Source: CAD feature listing. Evaluate the final solid. Frame: model axes, mm. Round coordinates to 2 decimals unless told otherwise and drop trailing zeros. Write each loop counter-clockwise with the first axis right and the second up, starting at its lowest first coordinate (ties: lowest second). Pieces come first, ordered by that corner, then holes. Notation, with made-up numbers: M 69.25,0.25 L 91.25,0.25 A25 ccw 91.25,27.25 Z; hole C 49.5,77 d8. An arc over 180 degrees is marked long. Use a Markdown table: item, result.
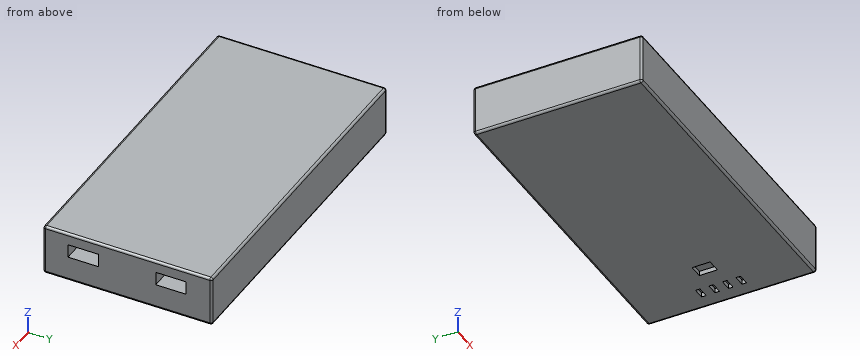
```python
from build123d import *

# Parameters (mm, degrees)
SKETCH_W        = 145
SKETCH_H        = 75
PAD_DEPTH       = 22.5
FILLET_R        = 1
SKETCH001_W     = 5
SKETCH001_H     = 2
SKETCH001_W_2   = 6
SKETCH001_H_2   = 8
POCKET_DEPTH    = 2
SKETCH002_W     = 13.5
SKETCH002_H     = 6
POCKET001_DEPTH = 20


with BuildPart() as part:
    # Sketch → Pad (new body)
    with BuildSketch(Plane.XY):
        Rectangle(SKETCH_W, SKETCH_H)
    extrude(amount=PAD_DEPTH)

    # Fillet
    fillet_edges = [part.edges().sort_by_distance(p)[0] for p in [
        (0, -37.5, 22.5),
        (72.5, 0, 22.5),
        (0, 37.5, 22.5),
        (-72.5, 0, 22.5),
        (-72.5, -37.5, 11.25),
        (72.5, -37.5, 11.25),
        (72.5, 37.5, 11.25),
        (72.5, 0, 0),
        (0, -37.5, 0),
        (0, 37.5, 0),
        (-72.5, 0, 0),
        (-72.5, 37.5, 11.25),
    ]]
    fillet(fillet_edges, radius=FILLET_R)

    # Sketch001 (on Face13 of Fillet) → Pocket (cut)
    with BuildSketch(Plane(origin=(0, 0, 0), x_dir=(1, 0, 0), z_dir=(0, 0, -1))):
        with Locations((63.084595, 9)):
            Rectangle(SKETCH001_W, SKETCH001_H)
        with Locations((63.084595, 3)):
            Rectangle(SKETCH001_W, SKETCH001_H)
        with Locations((63.084595, -3)):
            Rectangle(SKETCH001_W, SKETCH001_H)
        with Locations((63.084595, -9)):
            Rectangle(SKETCH001_W, SKETCH001_H)
        with Locations((49.584595, 0)):
            Rectangle(SKETCH001_W_2, SKETCH001_H_2)
    extrude(amount=-POCKET_DEPTH, mode=Mode.SUBTRACT)

    # Sketch002 (on Face12 of Pocket) → Pocket001 (cut)
    with BuildSketch(Plane.YZ.offset(72.5)):
        with Locations((19.25, 14.2)):
            Rectangle(SKETCH002_W, SKETCH002_H)
        with Locations((-19.75, 14.2)):
            Rectangle(SKETCH002_W, SKETCH002_H)
    extrude(amount=-POCKET001_DEPTH, mode=Mode.SUBTRACT)


solid = part.part
```
Q1. Section A-A on z = 13.75. Return loops of the section in (x, y), plus the area to 3 significant figures.
Results are:
| item | result |
|---|---|
| outline | M -72.5,-36.5 A1 ccw -71.5,-37.5 L 71.5,-37.5 A1 ccw 72.5,-36.5 L 72.5,-26.5 L 52.5,-26.5 L 52.5,-13 L 72.5,-13 L 72.5,12.5 L 52.5,12.5 L 52.5,26 L 72.5,26 L 72.5,36.5 A1 ccw 71.5,37.5 L -71.5,37.5 A1 ccw -72.5,36.5 Z |
| area | 10,300 mm^2 |
Q2. First-contact query: pin 1 Ø1.6 at (x, y) = (62.5, -3) entering from -Z; pin 2 Ø0.6 at (y, z) = (2, 0.5) entering from -X. Flat tips, straight axial feed; report the tip coordinate or a pass-through.
Results are:
| item | result |
|---|---|
| pin 1 | z = 2 |
| pin 2 | x = -72.48 |
Q3. Line query: L1, parallel to Y at x = 62, z = 15; L2, parallel to X at y = -20, z = 16. Output: solid intervals per line, ascending.
Results are:
| item | result |
|---|---|
| L1 | -37.5 to -26.5, -13 to 12.5, 26 to 37.5 |
| L2 | -72.5 to 52.5 |
Q4. Section C-C on y = -15.5. Return loops of the section in (x, z), plus the area to 3 significant figures.
Results are:
| item | result |
|---|---|
| outline | M -72.5,1 A1 ccw -71.5,0 L 71.5,0 A1 ccw 72.5,1 L 72.5,11.2 L 52.5,11.2 L 52.5,17.2 L 72.5,17.2 L 72.5,21.5 A1 ccw 71.5,22.5 L -71.5,22.5 A1 ccw -72.5,21.5 Z |
| area | 3,140 mm^2 |
Q5. Section B-B on x = 63. Give the number of separate pieces and of enclosed holes in the cut face, plus the area to 3 significant figures.
Results are:
| item | result |
|---|---|
| separate pieces | 1 |
| enclosed holes | 2 |
| area | 1,510 mm^2 |
